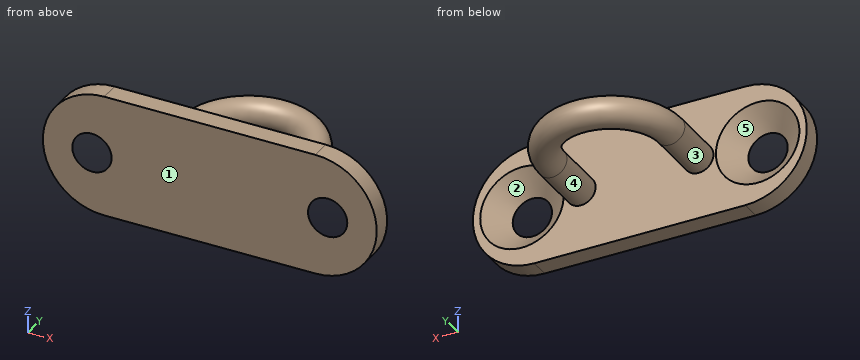
Autodesk Inventor part; units mm, degrees
ref_plane "cp1_XY" through (-12, 0, 0) normal (0, 1, 0) x (1, 0, 0)
ref_plane "cp1_YZ" through (-12, 0, 0) normal (1, 0, 0) x (0, 0, -1)
ref_plane "cp1_ZX" through (-12, 0, 0) normal (0, 0, -1) x (0, 1, 0)
sketch "Sketch_1" plane through (0, 0, 0) normal (0, 1, 0) x (-1, 0, 0)
  arc A0 (10.75, -6.25) -> (10.75, 6.25) centre (10.75, 0) ccw
  line L0 (10.75, 6.25) -> (-10.75, 6.25)
  arc A1 (-10.75, 6.25) -> (-10.75, -6.25) centre (-10.75, 0) ccw
  line L1 (-10.75, -6.25) -> (10.75, -6.25)
extrude "Extrusion1" add sketch "Sketch_1" along normal blind 2
sketch "Sketch_2" plane through (0, 2, 0) normal (0, 1, 0) x (1, 0, 0)
  circle A0 centre (-6, 0) radius 1.5
extrude "Extrusion2" add sketch "Sketch_2" along normal blind 5.5
sketch "Sketch_3" plane through (0, 2, 0) normal (0, 1, 0) x (1, 0, 0)
  circle A0 centre (6, 0) radius 1.5
extrude "Extrusion3" add sketch "Sketch_3" along normal blind 5.5
sketch "Sketch_4" plane through (0, 7.5, 0) normal (0, 1, 0) x (1, 0, 0)
  line L0 (0, 5) -> (0, -5)
  circle A0 centre (-6, 0) radius 1.5
revolve "Revolution1" add sketch "Sketch_4" angle 180 about axis through (0, 7.5, -5) along (0, 0, -1)
sketch "Sketch_5" plane through (0, 0, 0) normal (0, 0, 1) x (1, 0, 0)
  line L0 (-12, 0) -> (-12, 2)
  line L1 (-12, 2) -> (-7.75, 2)
  line L2 (-7.75, 2) -> (-10, 0)
  line L3 (-10, 0) -> (-12, 0)
  line L4 (-12, 0) -> (-12, 2)
revolve "Revolution2" cut sketch "Sketch_5" angle 360 about axis through (-12, 0, 0) along (0, -1, 0)
sketch "Sketch_7" plane through (0, 0, 0) normal (0, 0, 1) x (1, 0, 0)
  line L0 (12, 0) -> (12, 2)
  line L1 (12, 2) -> (16.25, 2)
  line L2 (16.25, 2) -> (14, 0)
  line L3 (14, 0) -> (12, 0)
  line L4 (12, 0) -> (12, 2)
revolve "Revolution3" cut sketch "Sketch_7" angle 360 about axis through (12, 0, 0) along (0, -1, 0)
ref_plane "cp1_XY" through (-12, 0, 0) normal (0, 1, 0) x (1, 0, 0)
ref_plane "cp1_YZ" through (-12, 0, 0) normal (1, 0, 0) x (0, 0, -1)
ref_plane "cp1_ZX" through (-12, 0, 0) normal (0, 0, -1) x (0, 1, 0)
ref_plane "cp2_XY" through (12, 0, 0) normal (0, 1, 0) x (1, 0, 0)
ref_plane "cp2_YZ" through (12, 0, 0) normal (1, 0, 0) x (0, 0, -1)
ref_plane "cp2_ZX" through (12, 0, 0) normal (0, 0, -1) x (0, 1, 0)
ref_plane "to_wire_XY" through (0, 13.5, 0) normal (1, 0, 0) x (0, 0, -1)
ref_plane "to_wire_YZ" through (0, 13.5, 0) normal (0, 0, -1) x (0, 1, 0)
ref_plane "to_wire_ZX" through (0, 13.5, 0) normal (0, 1, 0) x (1, 0, 0)
properties part number "TKCb"
Can you work these out from the model? Positions are in its coordinate system, mm. Face numbers are marked on the shaded views. A direction names the side the tool comes from. Round coordinates to 2 decimals unless told otherwise and drop trailing zeros. Write each loop counter-clockwise with the first axis right and the second up, starting at its lowest first coordinate (ties: lowest second). Pieces come first, ordered by that corner, then holes. Notation, with made-up numbers: (-4, 81.25) -> (14, 81.25) arc R21 ccw to (14, 99.25) -> close; hole circle Ø9 at (86, -14). An arc over 180 degrees is marked (long way). Use one line per item in the form item = value. Start each with the question number.
Q1. Imagine slicing it at B-B (x = -12). Please give me the cut outline in (y, z), then the cut area to 3 significant figures.
Q2. Which directions (+Z, -Z, +X, -X, +Y, -Y) give clear straight access to the entire face, cutting with the end or side of a thin tool? Please do the marked faces 4 and 5.
Q3. We'd pull the mould along Y, two halves only. Please class the marked faces 1, 2 and 3: +Y half, -Y half, draft (parallel to the pull), parting line (faces both ways), or undercut.
Q4. Imagine slicing it at A-A (z = 0.5). Count the separate pieces of the cut face and the enclosed holes in it, then the cut area to 3 significant figures.
Q5. If I drill on probe 1 along Y at (x, z) = (-4, -5.5); probe 2 along Z at (x, y) = (10, 1.25); probe 3 along X at (y, z) = (9.75, 0.25), over which ranges is the centre line in solid material (lowest first)? Write a range as [from, to].
Q6. I'm going to push flat-ended pins straight in: P1, Ø6, axis at y = 12, z = 1, coming from the -X side; P2, Ø5, axis at x = 5, z = 1, coming from the -Y side; P3, Ø3, axis at x = 1, z = -2.5, coming from the +Y side; P4, Ø5, axis at x = 11.5, z = 0, coming from the +Y side. Where does each tip first touch, or does it pass through?
Worked out:
q1.outline = (0, -6.12) -> (2, -6.12) -> (2, -4.25) -> (0, -2) -> close; (0, 2) -> (2, 4.25) -> (2, 6.12) -> (0, 6.12) -> close
q1.area = 12.0 mm^2
q2.face_4 = none
q2.face_5 = +Y
q3.face_1 = -Y half
q3.face_2 = +Y half
q3.face_3 = undercut
q4.separate_pieces = 3
q4.enclosed_holes = 1
q4.area = 128 mm^2
q5.probe_1 = [0, 2]
q5.probe_2 = [-6.25, -2.76], [2.76, 6.25]
q5.probe_3 = [-7.13, -3.92], [3.92, 7.13]
q6.P1 = -7.32
q6.P2 = 0
q6.P3 = 14.56
q6.P4 = 0.89
